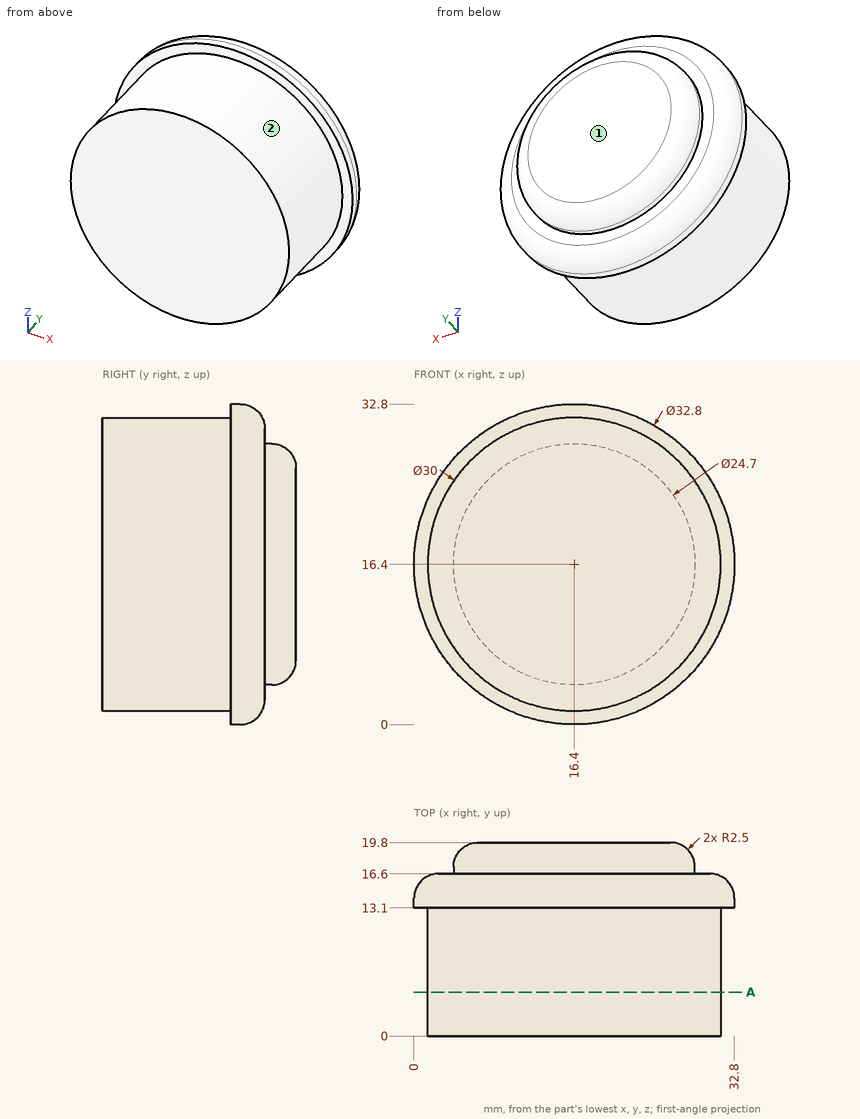
Here's the drawing with two shaded views (mm, measured from the low corner). I have some questions. A direction names the side the tool comes from. Round coordinates to 2 decimals unless told otherwise and drop trailing zeros. Loops run counter-clockwise (first coordinate to the right, second up) from the corner with the lowest first, then second, coordinate; pieces in that order, holes last.
Item 1: Please list where these lines run through material, in increasing order: L1, parallel to Y at x = 3.5, z = 18; L2, parallel to Y at x = 23, z = 24; L3, parallel to X at y = 14.75, z = 9.
Item 2: Will these pins go through, and if not, where does the flat tip stop? pin 1 Ø10 at (y, z) = (16.5, 9.5) entering from -X; pin 2 Ø1.5 at (x, z) = (6.5, 24.5) entering from +Y; pin 3 Ø1.5 at (y, z) = (16.5, 15) entering from +X.
Item 3: Suppose I cut it at A-A, the plane y = 4.5. Write out the boundary of the cut face in (x, z).
Item 4: Which directions (+Z, -Z, +X, -X, +Y, -Y) give clear straight access to the entire face, cutting with the end or side of a thin tool? Please do the marked faces 1 and 2.
Reported:
1. L1: y = 0 to 16.6
1. L2: y = 0 to 19.79
1. L3: x = 1.86 to 30.94
2. pin 1: stops at x = 0.19
2. pin 2: stops at y = 18.5
2. pin 3: stops at x = 32.12
3. outline: circle Ø30 at (16.4, 16.4)
4. face 1: +Z, -Z, +X, -X, +Y
4. face 2: -Y
